Autodesk Fusion 360 part; units mm, degrees
sketch "Sketch1" plane through (0, 0, 0) normal (0, 0, 1) x (1, 0, 0)
  line L0 (187.7997, -53.8565) -> (167.4907, -53.8666)
  line L1 (94.606, -62.0803) -> (77.4933, -62.0354)
  line L2 (160.6309, -126.1047) -> (174.4556, -134.0879)
  arc A0 (166.5198, -53.1058) -> (167.0103, -53.5064) centre (166.5198, -53.6063) cw
  arc A1 (167.4907, -53.8666) -> (167.0103, -53.5064) centre (167.4907, -53.3661) cw
  line L3 (166.5198, -53.1058) -> (149.4362, -53.1198)
  arc A2 (95.1065, -61.5798) -> (94.606, -62.0803) centre (94.6059, -61.5797) cw
  arc A3 (95.1081, -50.5552) -> (95.6086, -50.0547) centre (95.6086, -50.5552) cw
  line L4 (130.4348, -44.0784) -> (113.6387, -44.0918)
  line L5 (130.9353, -50.1013) -> (130.9353, -44.5789)
  line L6 (148.4352, -50.6175) -> (131.4358, -50.6018)
  line L7 (148.9357, -52.6194) -> (148.9357, -51.1179)
  line L8 (95.1081, -50.5552) -> (95.1065, -61.5798)
  line L9 (112.6549, -50.0547) -> (95.6086, -50.0547)
  line L10 (113.1383, -44.5922) -> (113.1554, -49.5542)
  arc A4 (113.1554, -49.5542) -> (112.6549, -50.0547) centre (112.6549, -49.5542) cw
  arc A5 (113.1383, -44.5922) -> (113.6387, -44.0918) centre (113.6387, -44.5923) cw
  arc A6 (130.4348, -44.0784) -> (130.9353, -44.5789) centre (130.4348, -44.5789) cw
  arc A7 (131.4358, -50.6018) -> (130.9353, -50.1013) centre (131.4358, -50.1013) cw
  arc A8 (148.4352, -50.6175) -> (148.9357, -51.1179) centre (148.4352, -51.1179) cw
  arc A9 (149.4362, -53.1198) -> (148.9357, -52.6194) centre (149.4362, -52.6193) cw
  arc A10 (187.7997, -53.8565) -> (188.3002, -54.357) centre (187.7997, -54.357) cw
  line L11 (94.2226, -113.6087) -> (143.2915, -121.3757)
  arc A11 (175.9364, -133.7828) -> (174.4556, -134.0879) centre (174.8961, -132.4797) cw
  line L12 (77.0866, -93.8666) -> (77.0866, -110.8501)
  line L13 (77.0357, -62.493) -> (77.0866, -76.7815)
  line L14 (188.3002, -54.357) -> (188.3943, -112.1213)
  line L15 (77.0866, -112.223) -> (77.0866, -110.8501)
  line L16 (77.0866, -76.7815) -> (77.0866, -93.8666)
  arc A12 (77.0357, -62.493) -> (77.4933, -62.0354) centre (77.4934, -62.493) cw
  line L17 (77.7476, -112.884) -> (94.2226, -113.6087)
  line L18 (143.2915, -121.3757) -> (160.6309, -126.1047)
  arc A13 (77.7476, -112.884) -> (77.0866, -112.223) centre (77.7476, -112.223) cw
  line L19 (175.9364, -133.7828) -> (188.3943, -112.1213)
  circle A14 centre (95.091, -66.866) radius 2.75
  circle A15 centre (95.091, -66.866) radius 1.75
  circle A16 centre (95.091, -83.9003) radius 2.75
  circle A17 centre (95.091, -83.9003) radius 1.75
  circle A18 centre (149.1137, -69.9169) radius 2.75
  circle A19 centre (149.1137, -69.9169) radius 1.75
  circle A20 centre (167.165, -110.4687) radius 2.75
  circle A21 centre (167.165, -110.4687) radius 1.75
  line L20 (177.5185, -135.0434) -> (190.3951, -112.6539)
  line L21 (190.3002, -54.3554) -> (190.3951, -112.6539)
  arc A22 (190.3002, -54.3554) -> (187.7992, -51.8565) centre (187.7997, -54.357) ccw
  line L22 (187.7992, -51.8565) -> (168.3155, -51.8662)
  arc A23 (168.3155, -51.8662) -> (166.519, -51.1058) centre (166.5198, -53.6063) ccw
  line L23 (166.519, -51.1058) -> (150.9357, -51.1186)
  line L24 (150.9357, -51.1186) -> (150.9357, -51.1179)
  arc A24 (150.9357, -51.1179) -> (148.4369, -48.6175) centre (148.4352, -51.1179) ccw
  line L25 (148.4369, -48.6175) -> (132.9353, -48.6032)
  line L26 (132.9353, -48.6032) -> (132.9353, -44.5789)
  arc A25 (132.9353, -44.5789) -> (130.434, -42.0784) centre (130.4348, -44.5789) ccw
  line L27 (130.434, -42.0784) -> (113.6379, -42.0918)
  arc A26 (113.6379, -42.0918) -> (111.1383, -44.6032) centre (113.6387, -44.5923) ccw
  line L28 (111.1383, -44.6032) -> (111.1502, -48.0547)
  line L29 (111.1502, -48.0547) -> (95.6086, -48.0547)
  arc A27 (95.6086, -48.0547) -> (93.1081, -50.5551) centre (95.6086, -50.5552) ccw
  line L30 (93.1081, -50.5551) -> (93.1067, -60.0763)
  line L31 (93.1067, -60.0763) -> (77.4982, -60.0354)
  arc A28 (77.4982, -60.0354) -> (75.0357, -62.5039) centre (77.4934, -62.493) ccw
  line L32 (75.0357, -62.5039) -> (75.0866, -76.785)
  line L33 (75.0866, -76.785) -> (75.0866, -93.8666)
  line L34 (75.0866, -93.8666) -> (75.0866, -110.8501)
  line L35 (75.0866, -112.223) -> (75.0866, -110.8501)
  arc A29 (75.0866, -112.223) -> (77.6889, -114.8834) centre (77.7476, -112.223) ccw
  line L36 (77.6889, -114.8834) -> (94.0216, -115.6018)
  line L37 (94.0216, -115.6018) -> (142.8708, -123.334)
  line L38 (142.8708, -123.334) -> (159.8549, -127.9661)
  line L39 (159.8549, -127.9661) -> (173.6348, -135.9234)
  arc A30 (173.6348, -135.9234) -> (177.5185, -135.0434) centre (174.8961, -132.4797) ccw
  line L40 (172.1905, -53.8642) -> (185.3472, -53.8642)
  line L41 (185.3472, -53.8642) -> (185.3472, -51.8577)
  line L42 (185.3472, -51.8577) -> (172.1905, -51.8577)
  line L43 (172.1905, -51.8577) -> (172.1905, -53.8642)
  point P0 (95.091, -83.9003)
  point P1 (149.1137, -69.9169)
  point P2 (167.165, -110.4687)
  dimension "d1" = 5.5
  dimension "d2" = 3.5
  dimension "d3" = 5.5
  dimension "d4" = 3.5
  dimension "d5" = 5.5
  dimension "d6" = 3.5
  dimension "d7" = 5.5
  dimension "d8" = 3.5
  dimension "d9" = -2
extrude "Extrude1" add sketch "Sketch1" along normal blind 1.5 contours L0 L1 L2 A0 A1 L3 A2 A3 L4 L5 L6 L7 L8 L9 L10 A4 A5 A6 A7 A8 A9 A10 L11 A11 L12 L13 L14 L15 L16 A12 L17 L18 A13 L19 L40 L41 makes body 1
extrude "Extrude2" add sketch "Sketch1" along normal blind 1 separate body contours A15 makes body 2
extrude "Extrude3" add sketch "Sketch1" along normal blind 1 separate body contours A17 makes body 3
extrude "Extrude4" add sketch "Sketch1" along normal blind 1 separate body contours A19 makes body 4
extrude "Extrude5" add sketch "Sketch1" along normal blind 1 separate body contours A21 makes body 5
extrude "Extrude6" add sketch "Sketch1" along normal blind 4 contours A14 bodies 1 2
extrude "Extrude7" add sketch "Sketch1" along normal blind 4 contours A16 bodies 1 3
extrude "Extrude8" add sketch "Sketch1" along normal blind 4 contours A18 bodies 1 4
extrude "Extrude9" add sketch "Sketch1" along normal blind 4 contours A20 bodies 1 5
extrude "Extrude10" add sketch "Sketch1" along normal blind 6 contours L0 L1 L2 A0 A1 L3 A2 A3 L4 L5 L6 L7 L8 L9 L10 A4 A5 A6 A7 A8 A9 A10 L11 A11 L12 L13 L14 L15 L16 A12 L17 L18 A13 L19 L20 L21 A22 L22 A23 L23 A24 L25 L26 A25 L27 A26 L28 L29 A27 L30 L31 A28 L32 L33 L34 L35 A29 L36 L37 L38 L39 A30 L41 L43 bodies 1
extrude "Extrude11" add sketch "Sketch1" along normal blind 3 contours L0 L22 L41 L43 bodies 1
chamfer "Chamfer1" distance 0.5 angle 45 1 edges at (92.5271, -82.9058, 1.5) on bodies 1
chamfer "Chamfer2" distance 0.5 angle 45 1 edges at (92.5271, -65.8715, 1.5) on bodies 1
chamfer "Chamfer3" distance 0.5 angle 45 1 edges at (146.5498, -68.9225, 1.5) on bodies 1
chamfer "Chamfer4" distance 0.5 angle 45 1 edges at (164.6011, -109.4743, 1.5) on bodies 1
Work out the finished part from the listing and answer in its coordinate system (mm). A direction names the side the tool comes from. Round coordinates to 2 decimals unless told otherwise and drop trailing zeros. Write each loop counter-clockwise with the first axis right and the second up, starting at its lowest first coordinate (ties: lowest second). Pieces come first, ordered by that corner, then holes. Notation, with made-up numbers: (3.5, -21) - (59.5, -21) arc R14 ccw to (59.5, -5) - close; hole circle Ø9 at (55, 12.5). An arc over 180 degrees is marked (long way). Return JSON: item names as keys, results as strings. Group by question number.
Q1. The part is cut by section C-C on x = 85.5. Write down the section's boundary in (y, z), then the cut area to 3 significant figures.
Q2. The part is cut by section B-B on y = -93.5. Write down the section's boundary in (x, z), then the cut area to 3 significant figures.
Q3. The part is cut by section A-A on x = 180. Write down the section's boundary in (y, z), then the cut area to 3 significant figures.
Q4. Find the intervals of material crossed by L1, parallel to X at y = -57.5, z = 5.1; L2, parallel to X at y = -94, z = 4.5; L3, parallel to Z at x = 91.5, y = -84.5, in increasing order.
Q5. The mould has two halves that part along X. Classify faces 1 (the flat face through (182.08, -123.1, 3.72)), 2 (the flat face through (103, -48.055, 3)), 3 (the flat face through (132, -88, 1.5)), 4 (the flat face through (118.104, -119.414, 2.958)): released by +X, released by -X, zero draft, split by the parting line, or undercut.
Q6. For faces 5 (the cylindrical face through (151.737, -70.743, 2.986)), 6 (the cylindrical face through (93.82, -48.81, 2.96)), determine the directions among +Z, -Z, +X, -X, +Y, -Y from which every point of the face is accessible in a straight line to the end or side of a thin tool.
Q7. Each of these flat-tipped pins is pushed along its axis until it touches: pin 1 Ø1.6 at (y, z) = (-52.5, 5) entering from +X; pin 2 Ø5 at (x, y) = (169.5, -103) entering from +Z; pin 3 Ø1 at (x, y) = (135, -77) entering from -Z; pin 4 Ø1 at (x, y) = (95, -67.5) entering from +Z. Where does it stop, or does it pass through?
Solved:
{
 "1": {"outline": "(-115.23, 0) - (-60.06, 0) - (-60.06, 6) - (-62.06, 6) - (-62.06, 1.5) - (-113.23, 1.5) - (-113.23, 6) - (-115.23, 6) - close", "area": "101 mm²"},
 "2": {"outline": "(75.09, 0) - (190.36, 0) - (190.36, 6) - (188.36, 6) - (188.36, 1.5) - (77.09, 1.5) - (77.09, 6) - (75.09, 6) - close", "area": "191 mm²"},
 "3": {"outline": "(-130.73, 0) - (-53.86, 0) - (-53.86, 1.5) - (-126.72, 1.5) - (-126.72, 6) - (-130.73, 6) - close; (-53.86, 0) - (-51.86, 0) - (-51.86, 3) - (-53.86, 3) - close", "area": "139 mm²"},
 "4": {"L1": "93.11 to 95.11, 188.31 to 190.31", "L2": "75.09 to 77.09, 188.36 to 190.36", "L3": "0 to 1.5"},
 "5": {"face 1": "undercut", "face 2": "zero draft", "face 3": "undercut", "face 4": "released by -X"},
 "6": {"face 5": "+Z", "face 6": "+Z, -Z, -X, +Y"},
 "7": {"pin 1": "x = 190.07", "pin 2": "z = 1.5", "pin 3": "z = 0", "pin 4": "z = 1"}
}
